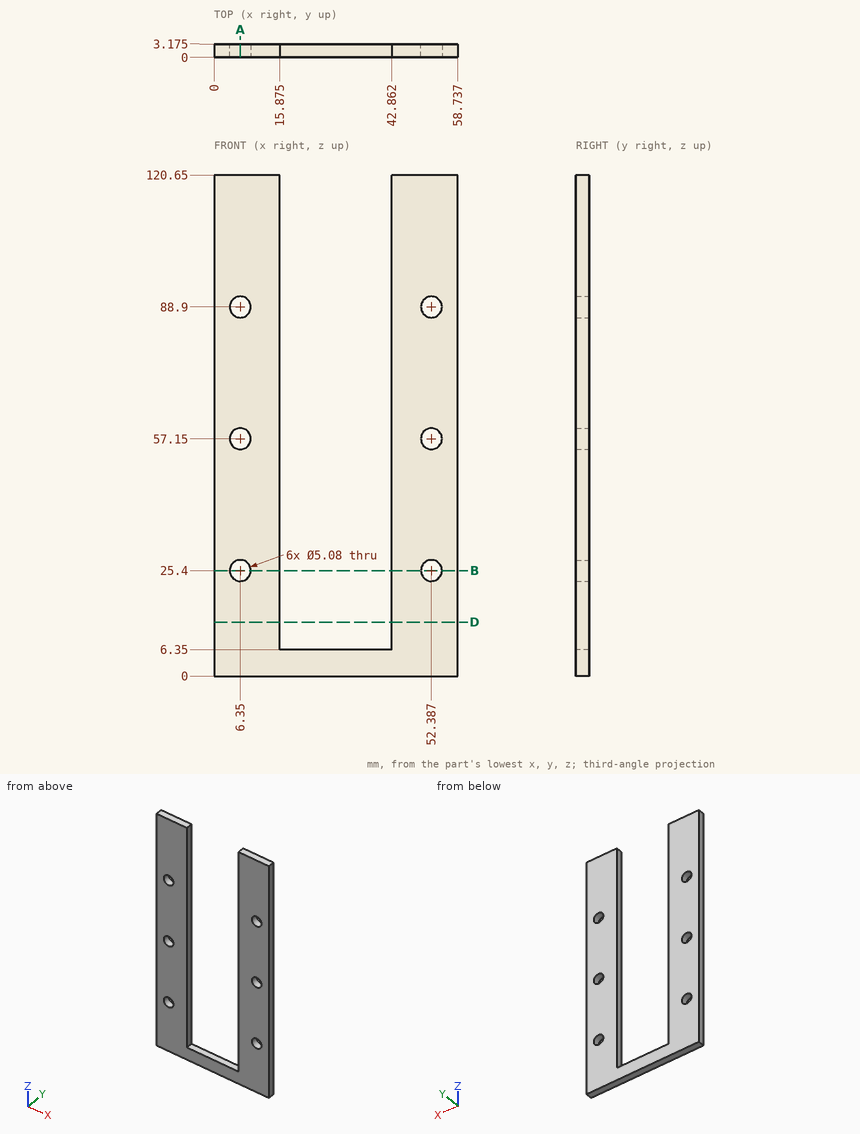
Check sheet for the drawn part. Datum: minimum x, y, z corner. Units: mm. Give positions to 0.01 mm unless a question says otherwise; leave off trailing zeros. Order: outer loops, then holes, each group sorted by start corner. A loop starts at its lowest first (then second) coordinate and runs counter-clockwise, first axis right, second up. Notation, with made-up numbers: (58, -33) - (87, -33) arc R14 ccw to (87, -12) - close; hole circle Ø9 at (85.5, 36.25). An arc over 180 degrees is marked (long way). Answer as a JSON object with one key per item and string values.
(1) Cross-section at D-D (z = 13). Record the cut outline in (x, y) (1 decimal).
Report:
{"outline": "(0, 0) - (15.9, 0) - (15.9, 3.2) - (0, 3.2) - close; (42.9, 0) - (58.7, 0) - (58.7, 3.2) - (42.9, 3.2) - close"}
(2) Material ranges on line 1 (Z direction, x = 6.35, y = 1.8); line 2 (X direction, y = 1.45, z = 88.9) (1 decimal); line 3 (X direction, y = 0.45, z = 19) (1 decimal), recorded low to high.
Report:
{"line 1": "0 to 22.86, 27.94 to 54.61, 59.69 to 86.36, 91.44 to 120.65", "line 2": "0 to 3.8, 8.9 to 15.9, 42.9 to 49.8, 54.9 to 58.7", "line 3": "0 to 15.9, 42.9 to 58.7"}
(3) Cross-section at B-B (z = 25.4). Record the cut outline in (x, y) (1 decimal).
Report:
{"outline": "(0, 0) - (3.8, 0) - (3.8, 3.2) - (0, 3.2) - close; (8.9, 0) - (15.9, 0) - (15.9, 3.2) - (8.9, 3.2) - close; (42.9, 0) - (49.8, 0) - (49.8, 3.2) - (42.9, 3.2) - close; (54.9, 0) - (58.7, 0) - (58.7, 3.2) - (54.9, 3.2) - close"}
(4) Cross-section at A-A (x = 6.35). State how many separate pieces and enclosed holes the cut face has.
Report:
{"separate pieces": "4", "enclosed holes": "0"}
